Geometry check sheet. Reference: drawing and pictorial views, mm from the part's lowest x, y, z. Coordinates: 2 decimals unless noted, no trailing zeros. Write each loop counter-clockwise with the first axis right and the second up, starting at its lowest first coordinate (ties: lowest second). Pieces come first, ordered by that corner, then holes. Notation, with made-up numbers: (-28, 70.25) - (-2, 70.25) arc R18 cw to (-2, 103.25) - close; hole circle Ø5 at (33, -33). An arc over 180 degrees is marked (long way). Use one line per item in the form item = value. Start each with the question number.
(1) Sectioned sample at D-D (x = 135). Record the cut outline in (y, z).
(2) Mould release check, pull along Z, two halves, no side actions. Record for the marked faces 1 and 2: released by +Z, released by -Z, zero draft, split by the parting line, or undercut.
(3) Sectioned sample at B-B (x = 195.5). Record the cut outline in (y, z).
(4) Sectioned sample at A-A (z = 2.5). Count the separate pieces of the cut face and the enclosed holes in it, and give its area (3 significant figures).
(5) Gauge pin test, flat end, axial feed: pin 1 Ø6.5 at (x, y) = (195.5, 20) entering from -Z. Record the tip position at first contact, or that the pin passes through.
(6) Material ranges on line 1 (Y direction, x = 175.5, z = 1.3); line 2 (Y direction, x = 154.5, z = 3.15), recorded low to high. Write a range as [from, to].
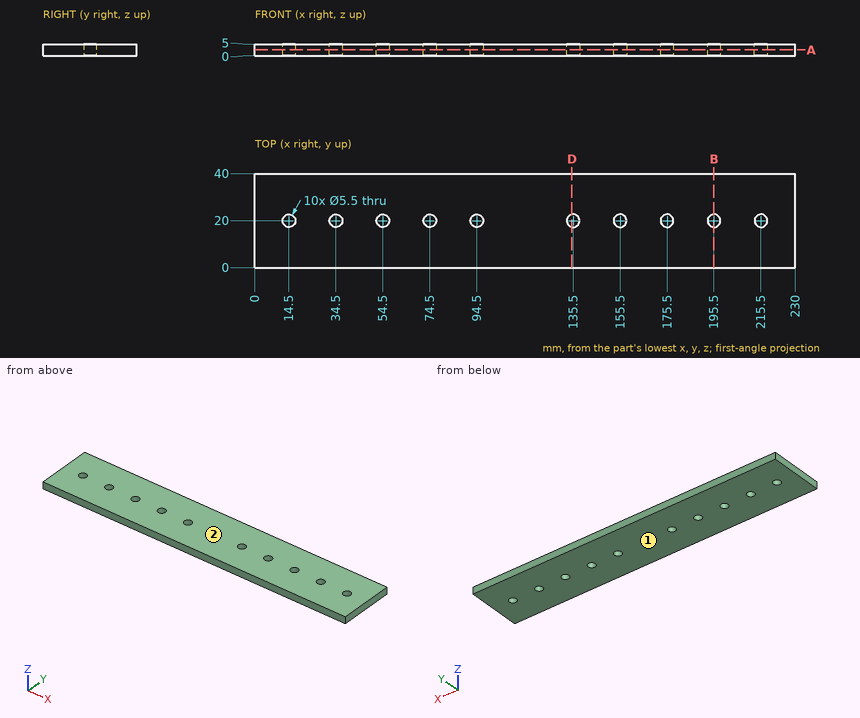
Answers below:
q1.outline = (0, 0) - (17.3, 0) - (17.3, 5) - (0, 5) - close; (22.7, 0) - (40, 0) - (40, 5) - (22.7, 5) - close
q2.face_1 = released by -Z
q2.face_2 = released by +Z
q3.outline = (0, 0) - (17.25, 0) - (17.25, 5) - (0, 5) - close; (22.75, 0) - (40, 0) - (40, 5) - (22.75, 5) - close
q4.separate_pieces = 1
q4.enclosed_holes = 10
q4.area = 8,960 mm2
q5.pin_1 = 0
q6.line_1 = [0, 17.25], [22.75, 40]
q6.line_2 = [0, 17.44], [22.56, 40]
